Build history of the part. All positions in model axes, mm. Coordinates: 2 decimals unless noted, no trailing zeros. Write each loop counter-clockwise with the first axis right and the second up, starting at its lowest first coordinate (ties: lowest second). Pieces come first, ordered by that corner, then holes.
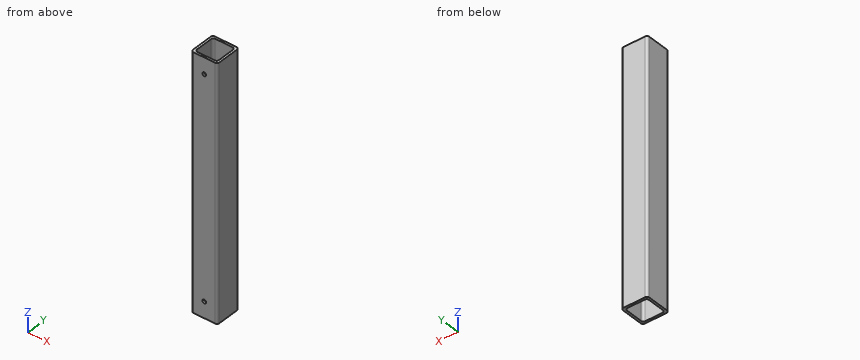
from build123d import *

# Parameters (mm, degrees)
BOSS_EXTRUDE1_DEPTH = 575
SKETCH2_R           = 8.5
CUT_EXTRUDE1_DEPTH  = 10


with BuildPart() as part:
    # Sketch1 → Boss-Extrude1 (new, symmetric)
    with BuildSketch(Plane.XY):
        with BuildLine():
            Line((-50, -60), (50, -60))
            ThreePointArc((50, -60), (57.071067812, -57.071067812), (60, -50))
            Line((60, -50), (60, 50))
            ThreePointArc((60, 50), (57.071067812, 57.071067812), (50, 60))
            Line((50, 60), (-50, 60))
            ThreePointArc((-50, 60), (-57.071067812, 57.071067812), (-60, 50))
            Line((-60, 50), (-60, -50))
            ThreePointArc((-60, -50), (-57.071067812, -57.071067812), (-50, -60))
        make_face()
        with BuildLine():
            Line((-40, -50), (40, -50))
            ThreePointArc((40, -50), (47.071067812, -47.071067812), (50, -40))
            Line((50, -40), (50, 40))
            ThreePointArc((50, 40), (47.071067812, 47.071067812), (40, 50))
            Line((40, 50), (-40, 50))
            ThreePointArc((-40, 50), (-47.071067812, 47.071067812), (-50, 40))
            Line((-50, 40), (-50, -40))
            ThreePointArc((-50, -40), (-47.071067812, -47.071067812), (-40, -50))
        make_face(mode=Mode.SUBTRACT)
    extrude(amount=BOSS_EXTRUDE1_DEPTH, both=True)

    # Sketch2 → Cut-Extrude1 (cut)
    with BuildSketch(Plane.XZ.offset(60)):
        with Locations(Location((0, 501, 0), (0, 0, 270))):
            Circle(SKETCH2_R)
        with Locations(Location((0, -501, 0), (0, 0, 90))):
            Circle(SKETCH2_R)
    extrude(amount=-CUT_EXTRUDE1_DEPTH, mode=Mode.SUBTRACT)


solid = part.part
(1) Slice it at A-A, the plane y = -23. List the corners of the cut face in (x, z).
(2) Probe L1, parallel to X at y = -21, z = -302; L2, parallel to X at y = 42, z = -215.5. List the from-to ranges inside material, lowest first.
(3) Slice it at C-C, the plane z = 264.5. List the corners of the cut face in (x, y).
Results:
1. outline: (-60, -575) - (-50, -575) - (-50, 575) - (-60, 575) - close; (50, -575) - (60, -575) - (60, 575) - (50, 575) - close
2. L1: x = -60 to -50, 50 to 60
2. L2: x = -60 to -49.8, 49.8 to 60
3. outline: (-60, -50) arc R10 ccw to (-50, -60) - (50, -60) arc R10 ccw to (60, -50) - (60, 50) arc R10 ccw to (50, 60) - (-50, 60) arc R10 ccw to (-60, 50) - close; hole (-50, -40) arc R10 ccw to (-40, -50) - (40, -50) arc R10 ccw to (50, -40) - (50, 40) arc R10 ccw to (40, 50) - (-40, 50) arc R10 ccw to (-50, 40) - close
